Autodesk Inventor part; units mm, degrees
ref_plane "YZ Plane" through (0, 0, 0) normal (1, 0, 0) x (0, 1, 0)
ref_plane "XZ Plane" through (0, 0, 0) normal (0, 1, 0) x (-1, 0, 0)
ref_plane "XY Plane" through (0, 0, 0) normal (0, 0, 1) x (1, 0, 0)
sketch "Sketch2" plane through (0, 0, 0) normal (0, 1, 0) x (-1, 0, 0)
  line L0 (0, 0) -> (5.881, 0)
  line L1 (5.881, 0) -> (5.881, 10)
  line L2 (5.881, 10) -> (0, 10)
  line L3 (0, 10) -> (0, 0)
  dimension "d2" = 5.881
  dimension "d3" = 10
extrude "Extrusion2" add sketch "Sketch2" along normal blind 1
sketch "Sketch3" plane through (0, 1, 0) normal (0, 1, 0) x (1, 0, 0)
  circle A0 centre (-2.9405, -5) radius 2.4
  dimension "d6" = 4.8
extrude "Extrusion3" cut sketch "Sketch3" against normal blind 1
sketch "Sketch4" plane through (0, 1, 0) normal (0, 1, 0) x (1, 0, 0)
  circle A0 centre (-2.9405, -5) radius 2.4
  line L0 (0, 0) -> (-5.881, 0)
  line L1 (-5.881, 0) -> (-5.881, -10)
  line L2 (-5.881, -10) -> (0, -10)
  line L3 (0, -10) -> (0, 0)
hole "Hole1" at (-2.881, 1, 1.3) direction (0, -1, 0) diameter 1.181 end through all
hole "Hole2" at (-2.881, 1, 8.7) direction (0, -1, 0) diameter 1.181 end through all
properties part number "recessedCoverslipHolder_v1"
Can you work these out from the model? Positions are in its coordinate system, mm. Round coordinates to 2 decimals unless told otherwise and drop trailing zeros. Loops run counter-clockwise (first coordinate to the right, second up) from the corner with the lowest first, then second, coordinate; pieces in that order, holes last. Notation, with made-up numbers: (20.5, 20.5) - (28.5, 20.5) arc R35 cw to (28.5, 55.5) - close; hole circle Ø2 at (65, 59). An arc over 180 degrees is marked (long way). Answer in a Markdown table with one row per item. Add a question column.
Q1. I want a section at D-D on y = 0.4. List the corners of the cut face in (x, z) for me.
Q2. We'd pull the mould along X, two halves only. Please class faces 1 (the flat face through (0, 0.5, 5.1)), 2 (the cylindrical face through (-1.65, 0.507, 2.976)), 3 (the flat face through (-2.9, 0.5, 0)): pulls with the +X half, pulls with the -X half, needs draft (parallel to the pull), parting line crosses it, or undercut.
Q3. I want a section at A-A on z = 5. List the corners of the cut face in (x, y) for me.
Q4. I want a section at B-B on x = -4.9. List the corners of the cut face in (y, z) for me.
Q5. I need wall thicknesses on L1, parallel to X at y = 0.75, z = 1.3; L2, parallel to Z at x = -3.2, y = 0.1; L3, parallel to X at y = 0.5, z = 5. Which ranges of each line are inside material? Lowest first, please.
Q6. I want a section at C-C on x = -3. List the corners of the cut face in (y, z) for me.
A:
| question | item | result |
|---|---|---|
| 1 | outline | (-5.88, 0) - (0, 0) - (0, 10) - (-5.88, 10) - close; hole circle Ø4.8 at (-2.94, 5); hole circle Ø1.18 at (-2.88, 1.3); hole circle Ø1.18 at (-2.88, 8.7) |
| 2 | face 1 | pulls with the +X half |
| 2 | face 2 | undercut |
| 2 | face 3 | needs draft |
| 3 | outline | (-5.88, 0) - (-5.34, 0) - (-5.34, 1) - (-5.88, 1) - close; (-0.54, 0) - (0, 0) - (0, 1) - (-0.54, 1) - close |
| 4 | outline | (0, 0) - (1, 0) - (1, 3.61) - (0, 3.61) - close; (0, 6.39) - (1, 6.39) - (1, 10) - (0, 10) - close |
| 5 | L1 | -5.88 to -3.47, -2.29 to 0 |
| 5 | L2 | 0 to 0.8, 1.8 to 2.61, 7.39 to 8.2, 9.2 to 10 |
| 5 | L3 | -5.88 to -5.34, -0.54 to 0 |
| 6 | outline | (0, 0) - (1, 0) - (1, 0.72) - (0, 0.72) - close; (0, 1.88) - (1, 1.88) - (1, 2.6) - (0, 2.6) - close; (0, 7.4) - (1, 7.4) - (1, 8.12) - (0, 8.12) - close; (0, 9.28) - (1, 9.28) - (1, 10) - (0, 10) - close |
